Autodesk Inventor part; units mm, degrees
ref_plane "YZ Plane" through (0, 0, 0) normal (1, 0, 0) x (0, 1, 0)
ref_plane "XZ Plane" through (0, 0, 0) normal (0, 1, 0) x (-1, 0, 0)
ref_plane "XY Plane" through (0, 0, 0) normal (0, 0, 1) x (1, 0, 0)
sketch "스케치1" plane through (0, 0, 0) normal (0, 0, 1) x (1, 0, 0)
  circle A0 centre (0, 0) radius 28.5
  line L0 (0, 20.304) -> (0, -24.0188)
  line L1 (-22.2174, 0) -> (23.7675, 0)
  circle A1 centre (0, 57) radius 7
  circle A2 centre (-49.6488, -28) radius 7
  circle A3 centre (49.6488, -28) radius 7
  arc A4 (13.8158, 65.0699) -> (-13.8158, 65.0699) centre (0, 57) ccw
  arc A5 (-63.4646, -19.9301) -> (-49.6488, -44) centre (-49.6488, -28) ccw
  arc A6 (49.6488, -44) -> (63.4646, -19.9301) centre (49.6488, -28) ccw
  line L2 (-13.8158, 65.0699) -> (-63.4646, -19.9301)
  line L3 (13.8158, 65.0699) -> (63.4646, -19.9301)
  line L4 (-49.6488, -44) -> (49.6488, -44)
  arc A7 (-52.7065, -21.7031) -> (-45.8423, -33.8746) centre (0, 0) ccw
  dimension "d0" = 57
  dimension "d4" = 14
  dimension "d6" = 14
  dimension "d7" = 28
  dimension "d8" = 32
  dimension "d9" = 32
  dimension "d10" = 32
extrude "돌출1" add sketch "스케치1" along normal blind 10
properties part number "240412_sketch2"
Input: part model. Units: mm. Frame: model coordinates. Give positions to 0.01 mm unless a question says otherwise; leave off trailing zeros. Order: outer loops, then holes, each group sorted by start corner. A loop starts at its lowest first (then second) coordinate and runs counter-clockwise, first axis right, second up.
1. Cut plane D-D (x = -46). Return loops of the section in (y, z), and give its area (3 significant figures).
Computed:
outline: (-44, 0) - (-33.97, 0) - (-33.97, 10) - (-44, 10) - close; (-22.03, 0) - (9.97, 0) - (9.97, 10) - (-22.03, 10) - close
area: 420 mm2
2. Cut plane C-C (y = 20). Return loops of the section in (x, z), and give its area (3 significant figures).
Computed:
outline: (-40.14, 0) - (-20.3, 0) - (-20.3, 10) - (-40.14, 10) - close; (20.3, 0) - (40.14, 0) - (40.14, 10) - (20.3, 10) - close
area: 397 mm2
3. Line query: probe 1 along Y at (x, z) = (0, 2.25); probe 2 along Y at (x, z) = (2.5, 0.75); probe 3 along Y at (x, z) = (-54, 5.5). Output: solid intervals per line, ascending.
Computed:
probe 1: y = -44 to -28.5, 28.5 to 50, 64 to 73
probe 2: y = -44 to -28.39, 28.39 to 50.46, 63.54 to 72.8
probe 3: y = -43.4 to -33.48, -22.52 to -3.73
4. Cut plane B-B (z = 3.25). Return loops of the section in (x, y).
Computed:
outline: (-63.46, -19.93) arc R16 ccw to (-49.65, -44) - (49.65, -44) arc R16 ccw to (63.46, -19.93) - (13.82, 65.07) arc R16 ccw to (-13.82, 65.07) - close; hole circle Ø14 at (-49.65, -28); hole circle Ø57 at (0, 0); hole circle Ø14 at (0, 57); hole circle Ø14 at (49.65, -28)
5. Pin query (flat end, axial travel): pin 1 Ø5 at (y, z) = (-24.5, 4.5) entering from +X; pin 2 Ø4 at (y, z) = (6.5, 6) entering from -X; pin 3 Ø3 at (x, y) = (-24.5, 51) entering from -Z; pin 4 Ø2 at (x, z) = (-27.5, 5) entering from +Y. Return the tip coordinate at first contact, or that it passes through.
Computed:
pin 1: stops at x = 65.62
pin 2: stops at x = -49.19
pin 3: passes through
pin 4: stops at y = 43.35
6. Draft query along Y for faces 1 (the face through (0, 73, 5)), 2 (the face through (26.327, 10.916, 4.93)), 3 (the face through (-1, -44, 5)), 4 (the face through (-0.91, 50.06, 4.93)). Return one class per face: released by +Y, released by -Y, zero draft, split by the parting line, or undercut.
Computed:
face 1: released by +Y
face 2: undercut
face 3: released by -Y
face 4: undercut
7. Cut plane A-A (x = 0). Return loops of the section in (y, z).
Computed:
outline: (-44, 0) - (-28.5, 0) - (-28.5, 10) - (-44, 10) - close; (28.5, 0) - (50, 0) - (50, 10) - (28.5, 10) - close; (64, 0) - (73, 0) - (73, 10) - (64, 10) - close
